```python
from build123d import *

# Parameters (mm, degrees)
SKETCH_7_W                  = 60
SKETCH_7_H                  = 64
EXTRUDE_1_DEPTH             = 10
SKETCH_12_R                 = 22.5
CUT_EXTRUDE_6_DEPTH         = 10
SKETCH_11_W                 = 69.759203198
SKETCH_11_H                 = 53.938344997
CUT_EXTRUDE_5_DEPTH         = 10
HOLE_WIZARD_M51_D           = 5.5
HOLE_WIZARD_M61_D           = 5
HOLE_WIZARD_M61_CSINK_D     = 7
HOLE_WIZARD_M61_CSINK_ANGLE = 90
CUT_EXTRUDE_7_DEPTH         = 4
FILLET_1_R                  = 2


with BuildPart() as part:
    # Эскиз7 → Бобышка-Вытянуть1 (new body)
    with BuildSketch(Plane(origin=(0, 0, 0), x_dir=(0, 0, -1), z_dir=(1, 0, 0))):
        with Locations((0, 2)):
            Rectangle(SKETCH_7_W, SKETCH_7_H)
    extrude(amount=EXTRUDE_1_DEPTH)

    # Эскиз12 → Вырез-Вытянуть6 (cut)
    with BuildSketch(Plane.ZY):
        Circle(SKETCH_12_R)
    extrude(amount=-CUT_EXTRUDE_6_DEPTH, mode=Mode.SUBTRACT)

    # Эскиз11 → Вырез-Вытянуть5 (cut)
    with BuildSketch(Plane(origin=(10, 0, 0), x_dir=(0, 0, -1), z_dir=(1, 0, 0))):
        with Locations((0.089558527, -7.969172499)):
            Rectangle(SKETCH_11_W, SKETCH_11_H)
    extrude(amount=-CUT_EXTRUDE_5_DEPTH, mode=Mode.SUBTRACT)

    # Сверло под метчик  спиральное M51 (through all)
    with Locations(Plane(origin=(10, 0, 0), x_dir=(0, 0, -1), z_dir=(1, 0, 0))):
        with Locations((-25, 25), (25, 25)):
            Hole(HOLE_WIZARD_M51_D / 2)

    # Отверстие обработанное метчиком M61 (through all)
    with Locations(Plane(origin=(0, 34, 0), x_dir=(1, 0, 0), z_dir=(0, 1, 0))):
        with Locations((5, 15), (5, -15)):
            CounterSinkHole(HOLE_WIZARD_M61_D / 2, HOLE_WIZARD_M61_CSINK_D / 2, counter_sink_angle=HOLE_WIZARD_M61_CSINK_ANGLE)

    # Эскиз16 → Вырез-Вытянуть7 (cut)
    with BuildSketch(Plane(origin=(10, 0, 0), x_dir=(0, 0, -1), z_dir=(1, 0, 0))):
        with BuildLine():
            Line((-25, 30), (-30, 30))
            Line((-30, 30), (-30, 19))
            Line((-30, 19), (-20, 19))
            Line((-20, 19), (-20, 25))
            ThreePointArc((-20, 25), (-21.464466094, 28.535533906), (-25, 30))
        make_face()
        with BuildLine():
            Line((20, 25), (20, 19))
            Line((20, 19), (30, 19))
            Line((30, 19), (30, 30))
            Line((30, 30), (25, 30))
            ThreePointArc((25, 30), (21.464466094, 28.535533906), (20, 25))
        make_face()
    extrude(amount=-CUT_EXTRUDE_7_DEPTH, mode=Mode.SUBTRACT)

    # Скругление1
    fillet_1_edges = [part.edges().sort_by_distance(p)[0] for p in [
        (3, 19, 30),
        (3, 19, -30),
    ]]
    fillet(fillet_1_edges, radius=FILLET_1_R)


solid = part.part
```
CAD build for the part. Positions are in the model's coordinates, mm. A direction names the side the tool comes from. Round coordinates to 2 decimals unless told otherwise and drop trailing zeros. Order: outer loops, then holes, each group sorted by start corner. A loop starts at its lowest first (then second) coordinate and runs counter-clockwise, first axis right, second up.
Item 1: Tool access for faces 4 (the face through (4, 19, 20)), 5 (the face through (8, 30, -28)): list every direction of +Z, -Z, +X, -X, +Y, -Y with a clear straight run to the whole face (end or side of a thin tool).
Item 2: Saw through at B-B on z = -15. Write the cut outline in (x, y), then the cut area to 3 significant figures.
Item 3: Saw through at D-D on z = 4.5. Write the cut outline in (x, y).
Item 4: Saw through at A-A on x = 5. Write the cut outline in (y, z), then the cut area to 3 significant figures.
Item 5: Pin check, flat tips, straight feed: pin 1 (2 mm diameter, centred on x = 7.5, y = 21, fed in from +Z); pin 2 (3 mm diameter, centred on x = 5, z = -15, fed in from -Y); pin 3 (1 mm diameter, centred on x = 6.5, z = -1.5, fed in from -Y); pin 4 (2 mm diameter, centred on x = 7.5, z = 28, fed in from -Y). Stop position of each tip, or through.
Item 6: Mould opens along Y. For faces 1 (the face through (3.04, 19.6, -29.43)), 2 (the face through (10, 28, 0)), 3 (the face through (2.958, 25.121, 22.253)) say: pulls with the +Y half, pulls with the -Y half, needs draft (parallel to the pull), parting line crosses it, or undercut.
Item 7: Probe line 1 along Z through (x, y) = (4.75, 28.25); line 2 along Y through (x, z) = (1.7, -25); line 3 along Z through (x, y) = (4, 24). List the from-to ranges inside material, lowest first.
Item 8: Saw through at C-C on z = 23. Write the cut outline in (x, y), then the cut area to 3 significant figures.
Reported:
1. face 4: +Z, -Z, +X, -X, -Y
1. face 5: -Z, +X, -Y
2. outline: (0, 19) - (2.5, 19) - (2.5, 33) - (1.5, 34) - (0, 34) - close; (7.5, 19) - (10, 19) - (10, 34) - (8.5, 34) - (7.5, 33) - close
2. area: 74.0 mm2
3. outline: (0, 22.05) - (10, 22.05) - (10, 34) - (0, 34) - close
4. outline: (19, -28) arc R2 ccw to (21, -30) - (34, -30) - (34, -18.5) - (33, -17.5) - (19, -17.5) - close; (19, -12.5) - (33, -12.5) - (34, -11.5) - (34, 11.5) - (33, 12.5) - (19, 12.5) - (19, 12.05) arc R22.5 cw to (19, -12.05) - close; (19, 17.5) - (33, 17.5) - (34, 18.5) - (34, 30) - (21, 30) arc R2 ccw to (19, 28) - close; hole circle Ø5.5 at (25, -25); hole circle Ø5.5 at (25, 25)
4. area: 642 mm2
5. pin 1: stops at z = 20
5. pin 2: passes through
5. pin 3: stops at y = 22.41
5. pin 4: stops at y = 30
6. face 1: pulls with the -Y half
6. face 2: needs draft
6. face 3: undercut
7. line 1: z = -30 to -17.49, -12.51 to 12.51, 17.49 to 30
7. line 2: y = 19 to 22.25, 27.75 to 34
7. line 3: z = -30 to -27.56, -22.44 to -17.29, -12.71 to 12.71, 17.29 to 22.44, 27.56 to 30
8. outline: (0, 19) - (6, 19) - (6, 23.11) - (0, 23.11) - close; (0, 26.89) - (6, 26.89) - (6, 29.58) - (10, 29.58) - (10, 34) - (0, 34) - close
8. area: 85.0 mm2
